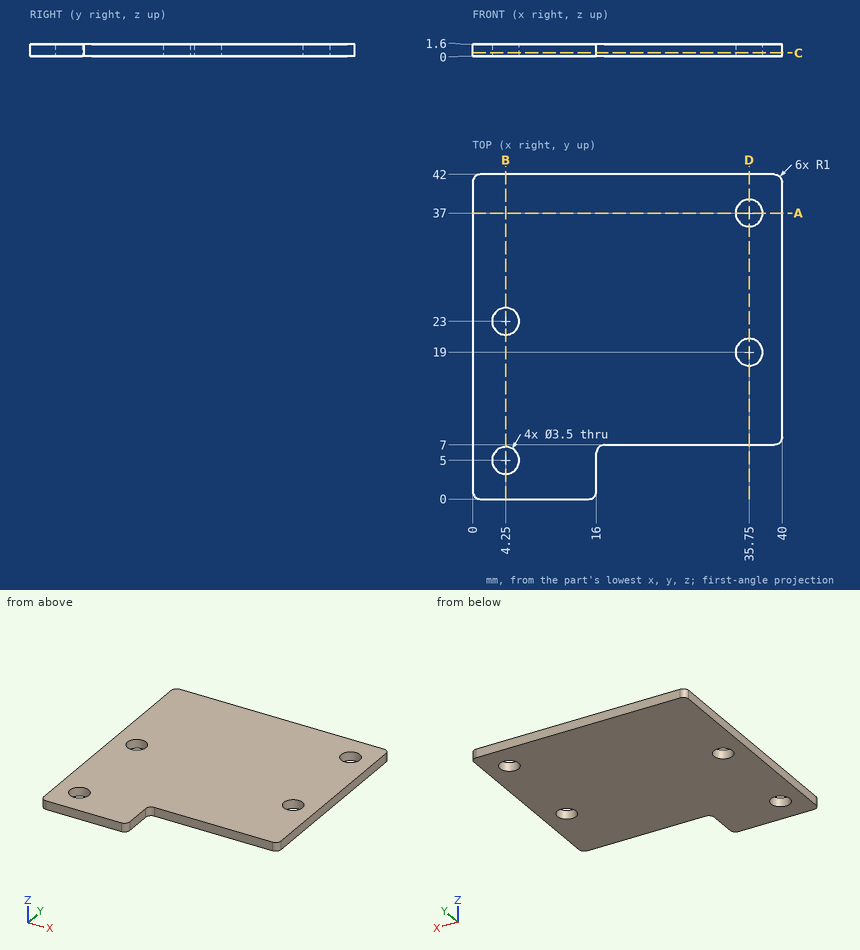
Design review of the part shown in the three views and the two pictorial views. Dimensions are in mm from the part's minimum x, y and z. Round coordinates to 2 decimals unless told otherwise and drop trailing zeros. Loops run counter-clockwise (first coordinate to the right, second up) from the corner with the lowest first, then second, coordinate; pieces in that order, holes last.
Q1. To check wall thickness, follow line 1 along Y through (x, z) = (35.75, 0.8); line 2 along Y through (x, z) = (4.25, 1.05); line 3 along X through (y, z) = (4, 0.4). State the ranges of each line that lie inside material, in increasing order.
Result sheet:
line 1: y = 7 to 17.25, 20.75 to 35.25, 38.75 to 42
line 2: y = 0 to 3.25, 6.75 to 21.25, 24.75 to 42
line 3: x = 0 to 2.81, 5.69 to 16
Q2. Add section B-B on x = 4.25. Write out the cut boundary in (y, z).
Result sheet:
outline: (0, 0) - (3.25, 0) - (3.25, 1.6) - (0, 1.6) - close; (6.75, 0) - (21.25, 0) - (21.25, 1.6) - (6.75, 1.6) - close; (24.75, 0) - (42, 0) - (42, 1.6) - (24.75, 1.6) - close
Q3. Insertion check: pin 1 Ø5.5 at (x, y) = (35.75, 19) entering from +Z; pin 2 Ø0.8 at (x, z) = (32, 0.5) entering from -Y. Each pin has a flat end and moves straight along its axis. Give the tip position at first contact, or say it passes through.
Result sheet:
pin 1: stops at z = 1.6
pin 2: stops at y = 7
Q4. Add section D-D on x = 35.75. Write out the cut boundary in (y, z).
Result sheet:
outline: (7, 0) - (17.25, 0) - (17.25, 1.6) - (7, 1.6) - close; (20.75, 0) - (35.25, 0) - (35.25, 1.6) - (20.75, 1.6) - close; (38.75, 0) - (42, 0) - (42, 1.6) - (38.75, 1.6) - close
Q5. Add section A-A on y = 37. Write out the cut boundary in (x, z).
Result sheet:
outline: (0, 0) - (34, 0) - (34, 1.6) - (0, 1.6) - close; (37.5, 0) - (40, 0) - (40, 1.6) - (37.5, 1.6) - close
Q6. Add section C-C on z = 0.45. Write out the cut boundary in (x, y).
Result sheet:
outline: (0, 1) arc R1 ccw to (1, 0) - (15, 0) arc R1 ccw to (16, 1) - (16, 6) arc R1 cw to (17, 7) - (39, 7) arc R1 ccw to (40, 8) - (40, 41) arc R1 ccw to (39, 42) - (1, 42) arc R1 ccw to (0, 41) - close; hole circle Ø3.5 at (4.25, 5); hole circle Ø3.5 at (4.25, 23); hole circle Ø3.5 at (35.75, 19); hole circle Ø3.5 at (35.75, 37)
